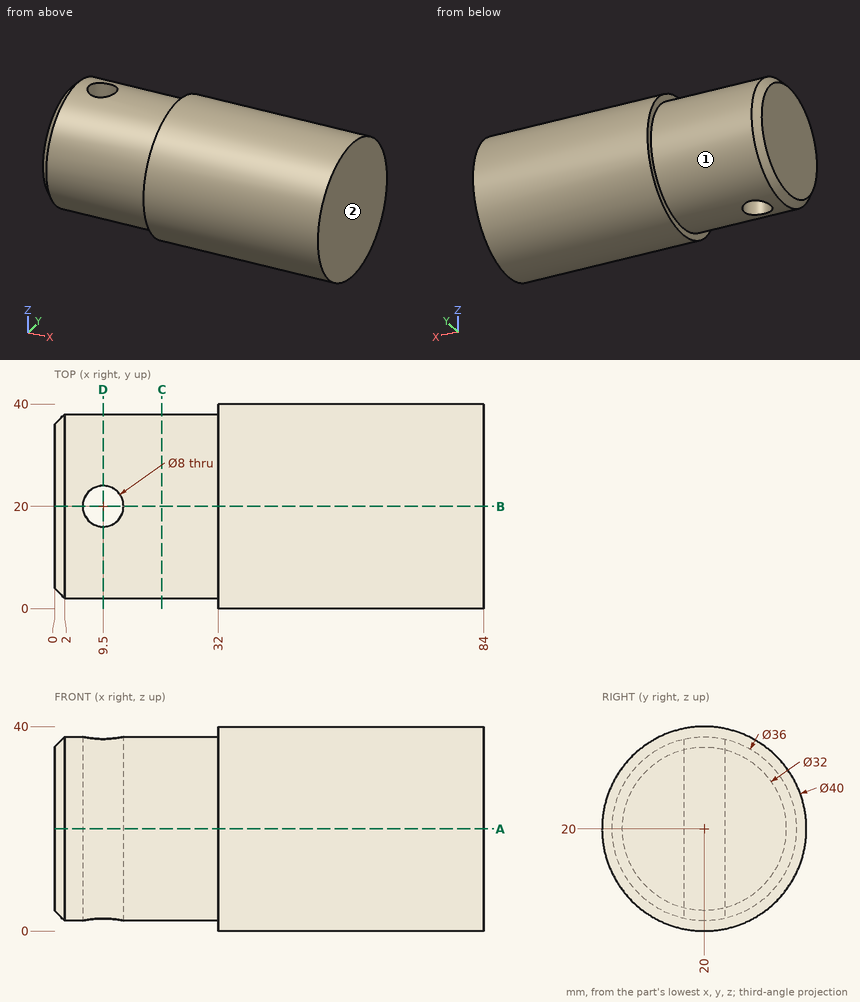
For this review, use the dimensioned drawing (mm, ordinates from the lowest corner) and the shaded views. A direction names the side the tool comes from. Round coordinates to 2 decimals unless told otherwise and drop trailing zeros. Order: outer loops, then holes, each group sorted by start corner. A loop starts at its lowest first (then second) coordinate and runs counter-clockwise, first axis right, second up. Notation, with made-up numbers: M -5.5,28 L 1.5,28 A22 cw 1.5,44 Z; hole C -22,-22 d5. An arc over 180 degrees is marked long. Use a Markdown table: item, result. Add a question column.
Item 1: Add section A-A, the plane z = 20. Give the boundary of the cut face in (x, y), then the cut area to 3 significant figures.
Item 2: Tool access review of the marked faces 1 and 2: name each direction out of +Z, -Z, +X, -X, +Y, -Y from which nothing blocks a thin tool from reaching the whole face with its end or side.
Item 3: Add section B-B, the plane y = 20. Give the boundary of the cut face in (x, z).
Item 4: To check wall thickness, follow line 1 along Y through (x, z) = (9.5, 19.5); line 2 along X through (y, z) = (20, 20); line 3 along X through (y, z) = (21, 37). State the ranges of each line that lie inside material, in increasing order.
Item 5: Add section C-C, the plane x = 21. Give the boundary of the cut face in (y, z), then the cut area to 3 significant figures.
Item 6: Add section D-D, the plane x = 9.5. Give the boundary of the cut face in (y, z).
Item 7: Insertion check: pin 1 (1.5 mm diameter, centred on x = 43.5, y = 35, fed in from -Z); pin 2 (12 mm diameter, centred on x = 57, y = 31, fed in from -Z); pin 3 (12 mm diameter, centred on x = 12, y = 25, fed in from -Z); pin 4 (7 mm diameter, centred on x = 9.5, y = 20, fed in from -Z). Each pin has a flat end and moves straight along its axis. Give the tip position at first contact, or say it passes through.
Geometry results:
| question | item | result |
|---|---|---|
| 1 | outline | M 0,4 L 2,2 L 32,2 L 32,0 L 84,0 L 84,40 L 32,40 L 32,38 L 2,38 L 0,36 Z; hole C 9.5,20 d8 |
| 1 | area | 3,180 mm² |
| 2 | face 1 | -X |
| 2 | face 2 | +Z, -Z, +X, +Y, -Y |
| 3 | outline | M 0,4 L 2,2 L 5.5,2 L 5.5,38 L 2,38 L 0,36 Z; M 13.5,2 L 32,2 L 32,0 L 84,0 L 84,40 L 32,40 L 32,38 L 13.5,38 Z |
| 4 | line 1 | y = 2.01 to 16, 24 to 37.99 |
| 4 | line 2 | x = 0 to 5.5, 13.5 to 84 |
| 4 | line 3 | x = 1.03 to 5.63, 13.37 to 84 |
| 5 | outline | C 20,20 d36 |
| 5 | area | 1,020 mm² |
| 6 | outline | M 16,2.45 L 16,37.55 A18 ccw Z; M 24,2.45 A18 ccw 24,37.55 Z |
| 7 | pin 1 | stops at z = 5.97 |
| 7 | pin 2 | stops at z = 0.64 |
| 7 | pin 3 | stops at z = 2 |
| 7 | pin 4 | passes through |
